from build123d import *

# Parameters (mm, degrees)
BOSS_EXTRUDE4_DEPTH  = 1.1
BOSS_EXTRUDE6_DEPTH  = 2
BOSS_EXTRUDE8_DEPTH  = 1
BOSS_EXTRUDE9_DEPTH  = 3.5
SKETCH13_W           = 4.301422626
SKETCH13_H           = 0.5
BOSS_EXTRUDE10_DEPTH = 0.5
BOSS_EXTRUDE11_DEPTH = 1.75


with BuildPart() as part:
    # Sketch1 → Boss-Extrude4 (new body)
    with BuildSketch(Plane(origin=(0, 0, 0), x_dir=(1, 0, 0), z_dir=(0, 1, 0))):
        Polygon((-13.958157374, 6.393603317), (4.779918737, 9.461645161), (7.776189987, 4.758788138), (7.776189987, -4.178449178), (-10.845876326, -4.178449178), align=None)
        Polygon((-12.039528162, 5.187772879), (-9.723810013, -2.678449178), (6.276189987, -2.678449178), (6.276189987, 4.321550822), (4.046279675, 7.821550822), align=None, mode=Mode.SUBTRACT)
    extrude(amount=BOSS_EXTRUDE4_DEPTH)

    # Sketch4 → Boss-Extrude6 (add)
    with BuildSketch(Plane(origin=(0, 1.1, 0), x_dir=(1, 0, 0), z_dir=(0, 1, 0))):
        Polygon((4.263894856, 7.479988594), (5.40328595, 8.483226777), (4.779918737, 9.461645161), (-13.958157374, 6.393603317), (-13.161594474, 3.687772879), (-11.597946778, 3.687772879), (-12.039528162, 5.187772879), (4.046279675, 7.821550822), align=None)
        Polygon((6.276189987, -0.978449178), (7.776189987, -0.978449178), (7.776189987, -4.178449178), (-10.845876326, -4.178449178), (-11.729039094, -1.178449178), (-10.165391397, -1.178449178), (-9.723810013, -2.678449178), (6.276189987, -2.678449178), align=None)
        Polygon((6.276189987, 2.258788138), (6.276189987, 4.321550822), (6.061258872, 4.658900219), (7.326319113, 5.464891898), (7.776189987, 4.758788138), (7.776189987, 2.258788138), align=None)
    extrude(amount=BOSS_EXTRUDE6_DEPTH)

    # Sketch8 → Boss-Extrude8 (add)
    with BuildSketch(Plane.XZ):
        Polygon((4.779918737, -9.461645161), (-13.958157374, -6.393603317), (-10.845876326, 4.178449178), (7.776189987, 4.178449178), (7.776189987, -4.758788138), align=None)
    extrude(amount=BOSS_EXTRUDE8_DEPTH)

    # Sketch12 → Boss-Extrude9 (add)
    with BuildSketch(Plane(origin=(0, 3.1, 0), x_dir=(1, 0, 0), z_dir=(0, 1, 0))):
        Polygon((-13.958157374, 6.393603317), (-8.037001115, 7.36309213), (-7.794628912, 5.882803065), (-12.039528162, 5.187772879), (-11.597946778, 3.687772879), (-13.161594474, 3.687772879), align=None)
    extrude(amount=BOSS_EXTRUDE9_DEPTH)

    # Sketch13 → Boss-Extrude10 (add)
    with BuildSketch(Plane(origin=(-1.141567738, 0, -6.972128883), x_dir=(0.9868593764655612, 0, -0.16158146886943345), z_dir=(0.16158146886943345, 0, 0.9868593764655612))):
        with Locations((-8.89236198, 6.35)):
            Rectangle(SKETCH13_W, SKETCH13_H)
    extrude(amount=BOSS_EXTRUDE10_DEPTH)

    # Sketch14 → Boss-Extrude11 (add)
    with BuildSketch(Plane.XZ.offset(1)):
        with BuildLine():
            Line((-12.435718696, -28.393603317), (-8.481738038, -27.756425594))
            Line((-8.481738038, -27.756425594), (-8.481738038, -32.756425594))
            Line((-8.481738038, -32.756425594), (-6.981738038, -32.756425594))
            Line((-6.981738038, -32.756425594), (-6.981738038, -27.514702969))
            Line((-6.981738038, -27.514702969), (11.853577786, -24.479421647))
            Line((11.853577786, -24.479421647), (11.853577786, -29.479421647))
            Line((11.853577786, -29.479421647), (13.353577786, -29.479421647))
            Line((13.353577786, -29.479421647), (13.353577786, -24.237699022))
            Line((13.353577786, -24.237699022), (17.18217535, -23.620726586))
            Line((17.18217535, -23.620726586), (16.863983568, -21.646200317))
            Line((16.863983568, -21.646200317), (6.843172004, -23.261038234))
            ThreePointArc((6.843172004, -23.261038234), (5.406002401, -22.709284639), (4.779918737, -21.302903559))
            Line((4.779918737, -21.302903559), (4.779918737, -9.461645161))
            Line((4.779918737, -9.461645161), (0.667895788, -8.788371214))
            ThreePointArc((0.667895788, -8.788371214), (2.057990663, -9.82529493), (2.779918737, -11.402125424))
            Line((2.779918737, -11.402125424), (2.779918737, -21.982368725))
            ThreePointArc((2.779918737, -21.982368725), (1.794986848, -23.340128824), (0.417030157, -24.296600818))
            Line((0.417030157, -24.296600818), (-7.469758325, -25.567544294))
            ThreePointArc((-7.469758325, -25.567544294), (-9.406227727, -25.006078343), (-10.378501991, -23.239771316))
            Line((-10.378501991, -23.239771316), (-10.378501991, -6.979711114))
            Line((-10.378501991, -6.979711114), (-13.958157374, -6.393603317))
            ThreePointArc((-13.958157374, -6.393603317), (-12.952521948, -7.628113726), (-12.435718696, -9.134179116))
            Line((-12.435718696, -9.134179116), (-12.435718696, -28.393603317))
        make_face()
    extrude(amount=-BOSS_EXTRUDE11_DEPTH)


solid = part.part
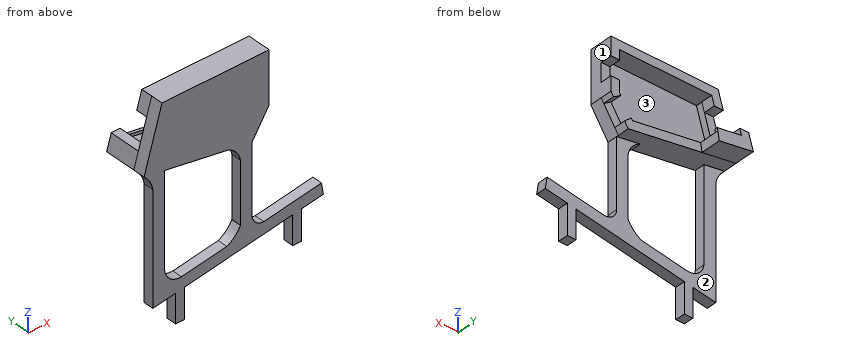
Here's how the part is built. I have some questions about the finished solid (model axes, mm). Face numbers are marked on the shaded views. Give positions to 0.01 mm unless a question says otherwise; leave off trailing zeros. Write each loop counter-clockwise with the first axis right and the second up, starting at its lowest first coordinate (ties: lowest second). Pieces come first, ordered by that corner, then holes. Notation, with made-up numbers: (-21, -5.75) -> (-14, -5.75) arc R18 cw to (-14, 29.25) -> close; hole circle Ø8 at (81.25, 23). An arc over 180 degrees is marked (long way). Use one line per item in the form item = value. Start each with the question number.
1. Imagine slicing it at D-D on z = -22.5. List the corners of the cut face in (x, y) for me.
2. Imagine slicing it at C-C on x = -6.5. List the corners of the cut face in (y, z) for me.
3. Imagine slicing it at B-B on y = 2.5. List the corners of the cut face in (x, z) for me, plus the area to 3 significant figures.
4. Thinking about a two-plate mould opening in X: for the marked faces 1, 2 and 3, which applies, +X half, -X half, draft (parallel to the pull), parting line (faces both ways), or undercut?
5. If I drill on L1, parallel to X at y = 0.25, z = -16.5; L2, parallel to Y at x = -1, z = -26.5; L3, parallel to Y at x = 6.5, z = -6, over which ranges is the centre line in solid material (lowest first)?
6. Will these pins go through, and if not, where does the flat tip stop? pin 1 Ø0.9 at (x, y) = (-2.5, 1.5) entering from -Z; pin 2 Ø1.4 at (y, z) = (-0.5, -12) entering from +X; pin 3 Ø8.5 at (x, z) = (-3.5, -2) entering from +Y.
7. Imagine slicing it at A-A on z = -17. List the corners of the cut face in (x, y) for me, plus the area to 3 significant figures.
Entries:
q1.outline = (-12.44, -1) -> (-10.38, -1) -> (-10.38, 0.75) -> (-12.44, 0.75) -> close; (2.48, -1) -> (5.21, -1) -> (5.21, 0.75) -> (2.48, 0.75) -> close; (11.57, -1) -> (17, -1) -> (17, 0.75) -> (11.57, 0.75) -> close
q2.outline = (-1, -27.44) -> (0.75, -27.44) -> (0.75, -25.41) -> (-1, -25.41) -> close; (-1, -7.61) -> (3.1, -7.61) -> (3.1, -6.09) -> (0, -6.09) -> (0, 2.68) -> (3.1, 2.68) -> (3.1, 4.18) -> (-1, 4.18) -> close
q3.outline = (-13.96, -6.39) -> (4.78, -9.46) -> (5.4, -8.48) -> (4.26, -7.48) -> (4.05, -7.82) -> (-12.04, -5.19) -> (-11.6, -3.69) -> (-13.16, -3.69) -> close; (-11.73, 1.18) -> (-10.17, 1.18) -> (-9.72, 2.68) -> (6.28, 2.68) -> (6.28, 0.98) -> (7.78, 0.98) -> (7.78, 4.18) -> (-10.85, 4.18) -> close; (6.06, -4.66) -> (7.33, -5.46) -> (7.78, -4.76) -> (7.78, -2.26) -> (6.28, -2.26) -> (6.28, -4.32) -> close
q3.area = 68.4 mm²
q4.face_1 = +X half
q4.face_2 = draft
q4.face_3 = undercut
q5.L1 = -12.44 to -10.38, 2.78 to 4.78
q5.L2 = -1 to 0.75
q5.L3 = -1 to 1.1
q6.pin_1 = -8.34
q6.pin_2 = 4.78
q6.pin_3 = 0
q7.outline = (-12.44, -1) -> (-10.38, -1) -> (-10.38, 0.75) -> (-12.44, 0.75) -> close; (2.78, -1) -> (4.78, -1) -> (4.78, 0.75) -> (2.78, 0.75) -> close
q7.area = 7.10 mm²
